Geometry check sheet. Reference: the model listing, model coordinates, mm. A direction names the side the tool comes from. Round coordinates to 2 decimals unless told otherwise and drop trailing zeros. Write each loop counter-clockwise with the first axis right and the second up, starting at its lowest first coordinate (ties: lowest second). Pieces come first, ordered by that corner, then holes. Notation, with made-up numbers: (-23.5, -37.75) - (-2.5, -37.75) arc R20 ccw to (-2.5, 1.25) - close; hole circle Ø4 at (58, 27). An arc over 180 degrees is marked (long way). One line per question, with ' | ' between items. Start each with the question number.
from build123d import *

# Parameters (mm, degrees)
SKIZZE1_W                        = 59
SKIZZE1_H                        = 59
AUFSATZ_LINEAR_AUSTRAGEN1_DEPTH  = 8
WANDUNG4_T                       = -2
SKIZZE5_W                        = 10
SKIZZE5_H                        = 10
AUFSATZ_LINEAR_AUSTRAGEN2_DEPTH  = 4
SKIZZE3_R                        = 1.6
SCHNITT_LINEAR_AUSTRAGEN8_DEPTH  = 10
SKIZZE6_W                        = 3.5
SKIZZE6_H                        = 10
SCHNITT_LINEAR_AUSTRAGEN10_DEPTH = 2
SCHNITT_LINEAR_AUSTRAGEN11_DEPTH = 3


with BuildPart() as part:
    # Skizze1 → Aufsatz-Linear austragen1 (new body)
    with BuildSketch(Plane.XY):
        Rectangle(SKIZZE1_W, SKIZZE1_H)
    extrude(amount=AUFSATZ_LINEAR_AUSTRAGEN1_DEPTH)

    # Wandung4
    wandung4_openings = [part.faces().sort_by_distance(p)[0] for p in [
        (0, 0, 0),
    ]]
    offset(amount=WANDUNG4_T, openings=wandung4_openings, kind=Kind.INTERSECTION)

    # Skizze5 → Aufsatz-Linear austragen2 (add)
    with BuildSketch(Plane(origin=(0, 0, 6), x_dir=(-1, 0, 0), z_dir=(0, 0, -1))):
        with Locations((-22.5, 22.5)):
            Rectangle(SKIZZE5_W, SKIZZE5_H)
        with Locations((22.5, 22.5)):
            Rectangle(SKIZZE5_W, SKIZZE5_H)
        with Locations((-22.5, -22.5)):
            Rectangle(SKIZZE5_W, SKIZZE5_H)
        with Locations((22.5, -22.5)):
            Rectangle(SKIZZE5_W, SKIZZE5_H)
    extrude(amount=AUFSATZ_LINEAR_AUSTRAGEN2_DEPTH)

    # Skizze3 → Schnitt-Linear austragen8 (cut)
    with BuildSketch(Plane.XY):
        with Locations((22.5, 22.5)):
            Circle(SKIZZE3_R)
        with Locations((-22.5, 22.5)):
            Circle(SKIZZE3_R)
        with Locations((-22.5, -22.5)):
            Circle(SKIZZE3_R)
        with Locations((22.5, -22.5)):
            Circle(SKIZZE3_R)
    extrude(amount=SCHNITT_LINEAR_AUSTRAGEN8_DEPTH, mode=Mode.SUBTRACT)

    # Skizze6 → Schnitt-Linear austragen10 (cut)
    with BuildSketch(Plane.ZY.offset(29.5)):
        with Locations((4.25, 4.5)):
            Rectangle(SKIZZE6_W, SKIZZE6_H)
    extrude(amount=-SCHNITT_LINEAR_AUSTRAGEN10_DEPTH, mode=Mode.SUBTRACT)

    # Skizze7 → Schnitt-Linear austragen11 (cut)
    with BuildSketch(Plane.XY.offset(8)):
        Polygon((-20.710214166, 25.6), (-24.289785834, 25.6), (-26.079571669, 22.5), (-24.289785834, 19.4), (-20.710214166, 19.4), (-18.920428331, 22.5), align=None)
        Polygon((24.237900311, 25.6), (20.658328642, 25.6), (18.868542808, 22.5), (20.658328642, 19.4), (24.237900311, 19.4), (26.027686146, 22.5), align=None)
        Polygon((-18.920428331, -22.5), (-20.710214166, -19.4), (-24.289785834, -19.4), (-26.079571669, -22.5), (-24.289785834, -25.6), (-20.710214166, -25.6), align=None)
        Polygon((24.289785834, -19.4), (20.710214166, -19.4), (18.920428331, -22.5), (20.710214166, -25.6), (24.289785834, -25.6), (26.079571669, -22.5), align=None)
    extrude(amount=-SCHNITT_LINEAR_AUSTRAGEN11_DEPTH, mode=Mode.SUBTRACT)


solid = part.part
Q1. Thickness scan on line 1 (Y direction, x = 22.5, z = 3.05); line 2 (Y direction, x = 5.5, z = 4.5). Record the ranges inside material, lowest first.
Q2. Section check B-B, the plane x = 22.5. Record the cut outline in (y, z), then the cut area to 3 significant figures.
Q3. Go/stop test with flat-tipped pins: P1, Ø5, axis at x = 22.5, y = 22.5, coming from the -Z side; P2, Ø8, axis at x = -19.5, y = -1, coming from the -Z side; P3, Ø1.9, axis at x = -22, y = -24, coming from the +Z side. Record where each tip stops, or that it passes through.
Q4. Section check A-A, the plane z = 3.5. Record the cut outline in (x, y), then the cut area to 3 significant figures.
Q5. Section check C-C, the plane y = 11.5. Record the cut outline in (x, z), then the cut area to 3 significant figures.
Q6. Draft check along Y on faces 1 (the flat face through (-29.5, 0, 2)), 2 (the flat face through (-22, 25.6, 7)). Enter one of: pulls with the +Y half, pulls with the -Y half, needs draft (parallel to the pull), parting line crosses it, or undercut.
Q7. Set-up check for faces 3 (the cylindrical face through (22.292, -20.914, 3.479)), 4 (the flat face through (-23, -25.6, 7)), 5 (the flat face through (17.5, -23, 4)): record each of +Z, -Z, +X, -X, +Y, -Y from which the full face is reachable in a straight line by a thin tool's end or side.
Result sheet:
1) line 1: -29.5 to -24.1, -20.9 to -17.5, 17.5 to 20.9, 24.1 to 29.5 | line 2: -29.5 to -27.5, 27.5 to 29.5
2) outline: (-29.5, 0) - (-27.5, 0) - (-27.5, 2) - (-24.1, 2) - (-24.1, 5) - (-25.6, 5) - (-25.6, 8) - (-29.5, 8) - close; (-20.9, 2) - (-17.5, 2) - (-17.5, 6) - (17.5, 6) - (17.5, 2) - (20.9, 2) - (20.9, 5) - (19.4, 5) - (19.4, 8) - (-19.4, 8) - (-19.4, 5) - (-20.9, 5) - close; (24.1, 2) - (27.5, 2) - (27.5, 0) - (29.5, 0) - (29.5, 8) - (25.6, 8) - (25.6, 5) - (24.1, 5) - close | area: 166 mm²
3) P1: z = 2 | P2: z = 6 | P3: z = 5
4) outline: (-29.5, -29.5) - (29.5, -29.5) - (29.5, 29.5) - (-29.5, 29.5) - (-29.5, 9.5) - (-27.5, 9.5) - (-27.5, 17.5) - (-17.5, 17.5) - (-17.5, 27.5) - (17.5, 27.5) - (17.5, 17.5) - (27.5, 17.5) - (27.5, -17.5) - (17.5, -17.5) - (17.5, -27.5) - (-17.5, -27.5) - (-17.5, -17.5) - (-27.5, -17.5) - (-27.5, -0.5) - (-29.5, -0.5) - close; hole circle Ø3.2 at (-22.5, -22.5); hole circle Ø3.2 at (-22.5, 22.5); hole circle Ø3.2 at (22.5, -22.5); hole circle Ø3.2 at (22.5, 22.5) | area: 804 mm²
5) outline: (-29.5, 0) - (-27.5, 0) - (-27.5, 6) - (27.5, 6) - (27.5, 0) - (29.5, 0) - (29.5, 8) - (-29.5, 8) - close | area: 142 mm²
6) face 1: needs draft | face 2: undercut
7) face 3: +Z, -Z | face 4: +Z | face 5: -Z
